Geometry: final body of the model. Coordinates: model frame, mm. Coordinates: 2 decimals unless noted, no trailing zeros. Order: outer loops, then holes, each group sorted by start corner. A loop starts at its lowest first (then second) coordinate and runs counter-clockwise, first axis right, second up. Notation, with made-up numbers: (43.5, 40) -> (60.5, 40) arc R10 cw to (60.5, 51) -> close; hole circle Ø7 at (30, 35). An arc over 180 degrees is marked (long way). Answer in a Markdown table with one row per item. Add a question column.
1) Section query B-B on y = 0.35. Count the separate pieces of the cut face and the enclosed holes in it, then the cut area to 3 significant figures.
2) Section query D-D on x = -24.5. Return the cut outline in (y, z).
3) Contact query for flat-ended pins moving along their axis: P1, Ø5.5, axis at x = -49.24, z = -27.7, coming from the +Y side; P2, Ø0.8, axis at x = -7.5, y = 1, coming from the -Z side. Output: stop coordinate, or through.
4) Section query A-A on x = -48. Return the cut outline in (y, z).
5) Section query C-C on z = -76.2. Return the cut outline in (x, y).
6) Ray query, line 1 (Z direction, x = 1.5, y = 1.3); line 2 (Z direction, x = -26, y = 1.3); line 3 (Z direction, x = -22, y = 1.1). Return the intervals inside material, ascending. Write a range as from..to.
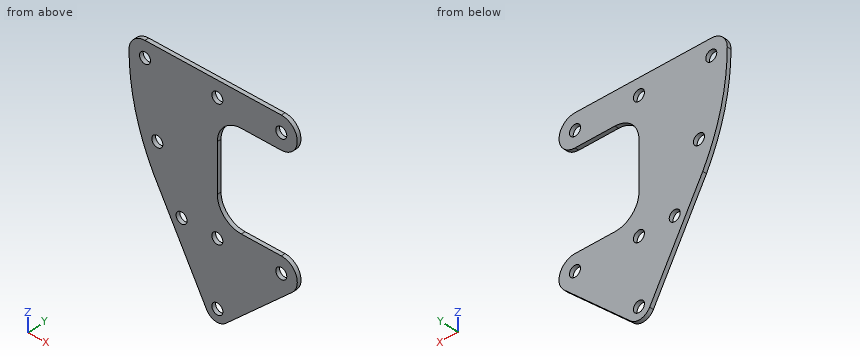
Autodesk Inventor part; units mm, degrees
ref_plane "YZ Plane" through (0, 0, 0) normal (1, 0, 0) x (0, 1, 0)
ref_plane "XZ Plane" through (0, 0, 0) normal (0, 1, 0) x (-1, 0, 0)
ref_plane "XY Plane" through (0, 0, 0) normal (0, 0, 1) x (1, 0, 0)
sketch "main" plane through (0, 0, 0) normal (0, 0, 1) x (1, 0, 0)
  line L0 (12.0188, -14.2552) -> (33.1027, 24.2387)
  circle A0 centre (21.9619, 13.8124) radius 2.1844
  circle A1 centre (31.5972, 36.5815) radius 2.1844
  circle A2 centre (36.4896, 64.2776) radius 2.1844
  line L1 (36.4904, 70.6276) -> (-17.6528, 70.6344)
  circle A3 centre (7.7473, 64.2844) radius 2.1844
  line L2 (7.7507, 48.4162) -> (7.7558, 29.3619)
  arc A4 (7.7507, 48.4162) -> (-1.7768, 57.9386) centre (-1.7743, 48.4136) ccw
  arc A5 (-1.7692, 19.8344) -> (7.7558, 29.3619) centre (-1.7692, 29.3594) ccw
  line L3 (-17.645, 57.9344) -> (-1.7768, 57.9386)
  arc A6 (-17.6528, 70.6344) -> (-17.645, 57.9344) centre (-17.645, 64.2844) ccw
  arc A7 (-17.6527, 19.8344) -> (-21.9541, 8.8131) centre (-17.6527, 13.4844) ccw
  circle A8 centre (7.7473, 13.4844) radius 2.1844
  line L4 (-1.7692, 19.8344) -> (-17.6527, 19.8344)
  arc A9 (4.4483, -15.4983) -> (12.0188, -14.2552) centre (7.7473, -11.9156) ccw
  line L5 (4.4483, -15.4983) -> (-21.9541, 8.8131)
  circle A10 centre (7.7473, -11.9156) radius 2.1844
  circle A11 centre (-17.645, 64.2844) radius 2.1844
  circle A12 centre (-17.6527, 13.4844) radius 2.1844
  arc A13 (42.8396, 64.2776) -> (36.4904, 70.6276) centre (36.4896, 64.2776) ccw
  arc A14 (33.1027, 24.2387) -> (42.8396, 64.2776) centre (-44.3506, 64.2776) ccw
  point P0 (10.5119, 26.5593)
  dimension "d1" = 9.7405
  dimension "d2" = 4.3688
  dimension "d3" = 4.3688
  dimension "d4" = 4.3688
  dimension "d5" = 4.3688
  dimension "d6" = 4.3688
  dimension "d10" = 50.8
  dimension "d11" = 50.8
  dimension "d13" = 6.35
sketch "Sketch1" plane through (0, 0, 0) normal (0, 1, 0) x (-1, 0, 0)
  line L0 (29.6638, -78.5396) -> (50.7478, -40.0457)
  circle A0 centre (39.607, -50.472) radius 2.1844
  circle A1 centre (49.2422, -27.7029) radius 2.1844
  circle A2 centre (54.1346, -0.0068) radius 2.1844
  line L1 (54.1354, 6.3432) -> (-0.0077, 6.35)
  circle A3 centre (25.3923, 0) radius 2.1844
  line L2 (25.3957, -15.8682) -> (25.4009, -34.9224)
  arc A4 (25.3957, -15.8682) -> (15.8682, -6.3457) centre (15.8707, -15.8707) ccw
  arc A5 (15.8759, -44.45) -> (25.4009, -34.9224) centre (15.8759, -34.925) ccw
  line L3 (0, -6.35) -> (15.8682, -6.3457)
  arc A6 (-0.0077, 6.35) -> (0, -6.35) centre (0, 0) ccw
  arc A7 (-0.0077, -44.45) -> (-4.309, -55.4713) centre (-0.0077, -50.8) ccw
  circle A8 centre (25.3923, -50.8) radius 2.1844
  line L4 (15.8759, -44.45) -> (-0.0077, -44.45)
  arc A9 (22.0933, -79.7827) -> (29.6638, -78.5396) centre (25.3923, -76.2) ccw
  line L5 (22.0933, -79.7827) -> (-4.309, -55.4713)
  circle A10 centre (25.3923, -76.2) radius 2.1844
  circle A11 centre (0, 0) radius 2.1844
  circle A12 centre (-0.0077, -50.8) radius 2.1844
  arc A13 (60.4846, -0.0068) -> (54.1354, 6.3432) centre (54.1346, -0.0068) ccw
  arc A14 (50.7478, -40.0457) -> (60.4846, -0.0068) centre (-26.7056, -0.0068) ccw
extrude "Extrusion1" add sketch "Sketch1" along normal blind 1.5875
properties part number "Funnel Gusset Back Improved V2" material "Acetal Resin, White"
Result:
| question | item | result |
|---|---|---|
| 1 | separate pieces | 1 |
| 1 | enclosed holes | 8 |
| 1 | area | 3,120 mm2 |
| 2 | outline | (0, -80.99) -> (1.59, -80.99) -> (1.59, -78.19) -> (0, -78.19) -> close; (0, -74.21) -> (1.59, -74.21) -> (1.59, -52.79) -> (0, -52.79) -> close; (0, -48.81) -> (1.59, -48.81) -> (1.59, -38.97) -> (0, -38.97) -> close; (0, -11.84) -> (1.59, -11.84) -> (1.59, -1.99) -> (0, -1.99) -> close; (0, 1.99) -> (1.59, 1.99) -> (1.59, 6.35) -> (0, 6.35) -> close |
| 3 | P1 | y = 1.59 |
| 3 | P2 | z = -66.71 |
| 4 | outline | (0, -45.06) -> (1.59, -45.06) -> (1.59, -29.5) -> (0, -29.5) -> close; (0, -25.91) -> (1.59, -25.91) -> (1.59, 6.34) -> (0, 6.34) -> close |
| 5 | outline | (-30.95, 0) -> (-27.58, 0) -> (-27.58, 1.59) -> (-30.95, 1.59) -> close; (-23.21, 0) -> (-18.2, 0) -> (-18.2, 1.59) -> (-23.21, 1.59) -> close |
| 6 | line 1 | -58.06..-52.4, -49.2..-44.63, -6.17..-1.59, 1.59..6.17 |
| 6 | line 2 | -81.03..-78.3, -74.1..-52.9, -48.7..-2.1, 2.1..6.35 |
| 6 | line 3 | -79.7..-42.22, -8.58..6.35 |
